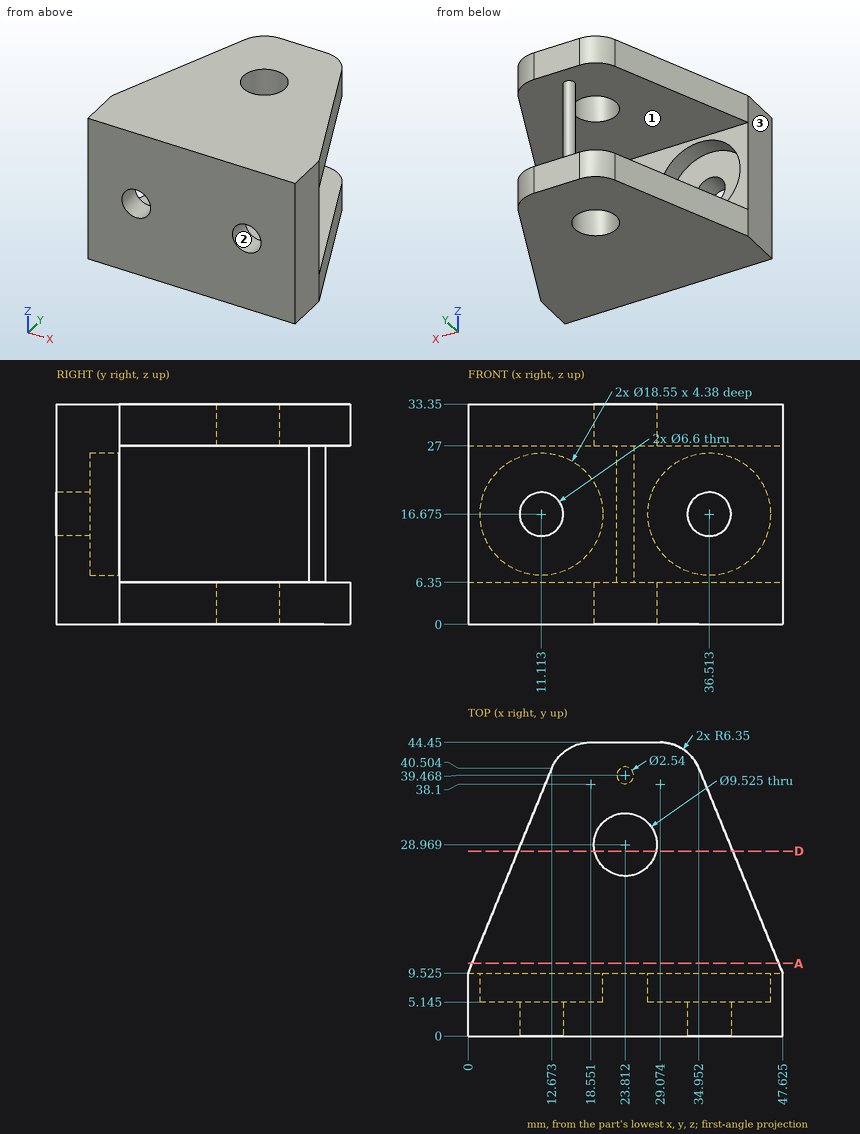
Verification items for this drawing (mm, ordinates from the low corner). Round coordinates to 2 decimals unless told otherwise and drop trailing zeros. Order: outer loops, then holes, each group sorted by start corner. A loop starts at its lowest first (then second) coordinate and runs counter-clockwise, first axis right, second up. Notation, with made-up numbers: (-21.75, -32) - (20.25, -32) arc R22 ccw to (20.25, -13) - close; hole circle Ø8 at (-11.5, 2). An arc over 180 degrees is marked (long way). Use CSV: the item, a comma, the result in double quotes.
(1) Mould release check, pull along X, two halves, no side actions. Record for the marked faces 1, 2 and 3: released by +X, released by -X, zero draft, split by the parting line, or undercut.
Entries:
face 1,"zero draft"
face 2,"undercut"
face 3,"released by -X"
(2) Gauge pin test, flat ends, axial feed: pin 1 Ø6 at (y, z) = (35, 29.5) entering from -X (1 decimal); pin 2 Ø5.5 at (x, z) = (11.5, 20.5) entering from +Y (1 decimal); pin 3 Ø12 at (y, z) = (20, 9) entering from +X. Record the tip position at first contact, or that the pin passes through.
Entries:
pin 1,"x = 9.2"
pin 2,"y = 5.1"
pin 3,"x = 45.54"
(3) Section check A-A on y = 11. Record the boundary of the cut face in (x, z).
Entries:
outline,"(0.6, 0) - (47.02, 0) - (47.02, 6.35) - (0.6, 6.35) - close; (0.6, 27) - (47.02, 27) - (47.02, 33.35) - (0.6, 33.35) - close"
(4) Thickness scan on probe 1 along Z at (x, y) = (32, 24); probe 2 along X at (y, z) = (9, 19.5) (1 decimal); probe 3 along Y at (x, z) = (39, 24) (1 decimal). Record the ranges inside material, lowest first. Write a range as from..to.
Entries:
probe 1,"0..6.35, 27..33.35"
probe 2,"0..2.3, 19.9..27.7, 45.3..47.6"
probe 3,"0..5.1"
(5) Section check D-D on y = 28. State how many separate pieces and enclosed holes the cut face has.
Entries:
separate pieces,"4"
enclosed holes,"0"
